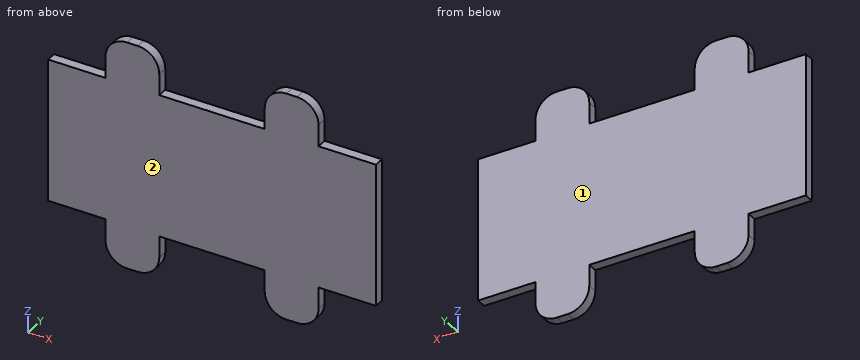
from build123d import *

# Parameters (mm, degrees)
F1_DEPTH = 0.7
F2_R     = 1.5


with BuildPart() as f1:
    # F0 (on Front) → F1 (new body)
    with BuildSketch(Plane.XZ):
        Polygon((3.75, -3), (3.75, 0), (11.1, 0), (11.1, -3), (14.85, -3), (14.85, 0), (18.85, 0), (18.85, 10), (14.85, 10), (14.85, 13), (11.1, 13), (11.1, 10), (3.75, 10), (3.75, 13), (0, 13), (0, 10), (-4, 10), (-4, 0), (0, 0), (0, -3), align=None)
    extrude(amount=F1_DEPTH)

    # F2
    f2_edges = [f1.edges().sort_by_distance(p)[0] for p in [
        (0, -0.35, 13),
        (3.75, -0.35, 13),
        (11.1, -0.35, 13),
        (14.85, -0.35, 13),
        (0, -0.35, -3),
        (3.75, -0.35, -3),
        (11.1, -0.35, -3),
        (14.85, -0.35, -3),
    ]]
    fillet(f2_edges, radius=F2_R)


solid = f1.part
The listing builds one solid part. Answer for the finished solid, in the listing's coordinates (mm). Face numbers are marked on the shaded views. Round coordinates to 2 decimals unless told otherwise and drop trailing zeros. Write each loop counter-clockwise with the first axis right and the second up, starting at its lowest first coordinate (ties: lowest second). Pieces come first, ordered by that corner, then holes. Notation, with made-up numbers: (43, 22.5) - (72, 22.5) arc R7 cw to (72, 30.5) - close; hole circle Ø4 at (50.5, 40.25). An arc over 180 degrees is marked (long way). Use a Markdown table: item, result. Add a question column.
1. For a pull along Y with two mould halves and no side action, classify the marked faces 1 and 2 as +Y half, -Y half, draft (parallel to the pull), parting line (faces both ways), or undercut.
2. The part is cut by section B-B (y = -0.5). Write down the section's boundary in (x, z), and give its area (3 significant figures).
3. The part is cut by section D-D (x = 14). Write down the section's boundary in (y, z), and give its area (3 significant figures).
4. Consider line 1 (X direction, y = -0.15, z = 11.5); line 2 (Z direction, x = -2.25, y = -0.2). Determine where each line is inside the solid, lowest interval first.
5. The part is cut by section C-C (x = 5). Write down the section's boundary in (y, z), and give its area (3 significant figures).
6. The part is cut by section A-A (z = -0.75). Write down the section's boundary in (x, y).
Reported:
| question | item | result |
|---|---|---|
| 1 | face 1 | +Y half |
| 1 | face 2 | -Y half |
| 2 | outline | (-4, 0) - (0, 0) - (0, -1.5) arc R1.5 ccw to (1.5, -3) - (2.25, -3) arc R1.5 ccw to (3.75, -1.5) - (3.75, 0) - (11.1, 0) - (11.1, -1.5) arc R1.5 ccw to (12.6, -3) - (13.35, -3) arc R1.5 ccw to (14.85, -1.5) - (14.85, 0) - (18.85, 0) - (18.85, 10) - (14.85, 10) - (14.85, 11.5) arc R1.5 ccw to (13.35, 13) - (12.6, 13) arc R1.5 ccw to (11.1, 11.5) - (11.1, 10) - (3.75, 10) - (3.75, 11.5) arc R1.5 ccw to (2.25, 13) - (1.5, 13) arc R1.5 ccw to (0, 11.5) - (0, 10) - (-4, 10) - close |
| 2 | area | 270 mm^2 |
| 3 | outline | (-0.7, -2.85) - (0, -2.85) - (0, 12.85) - (-0.7, 12.85) - close |
| 3 | area | 11.0 mm^2 |
| 4 | line 1 | 0 to 3.75, 11.1 to 14.85 |
| 4 | line 2 | 0 to 10 |
| 5 | outline | (-0.7, 0) - (0, 0) - (0, 10) - (-0.7, 10) - close |
| 5 | area | 7.00 mm^2 |
| 6 | outline | (0, -0.7) - (3.75, -0.7) - (3.75, 0) - (0, 0) - close; (11.1, -0.7) - (14.85, -0.7) - (14.85, 0) - (11.1, 0) - close |
